The listing builds one solid part. Answer for the finished solid, in the listing's coordinates (mm). A direction names the side the tool comes from. Coordinates: 2 decimals unless noted, no trailing zeros. Write each loop counter-clockwise with the first axis right and the second up, starting at its lowest first coordinate (ties: lowest second). Pieces come first, ordered by that corner, then holes. Notation, with made-up numbers: M 58,17 L 79,17 A22 cw 79,42 Z; hole C -26.75,71.25 d4. An arc over 180 degrees is marked long. Write item = value, one per line. Start each with the question number.
```python
from build123d import *

# Parameters (mm, degrees)
F1_DEPTH = 6.35
F3_DEPTH = 2.54


with BuildPart() as f1:
    # F0 (on Top) → F1 (new body)
    with BuildSketch(Plane.XY):
        Polygon((-19.068402, 7.360227), (-42.225117, 7.360227), (-57.954384, -14.267517), (-20.852379, -14.267517), (-20.852379, -24.618464), (10.865408, -24.618464), (10.865408, -14.267517), (39.400437, -14.267517), (52.040033, 7.360227), (12.264185, 7.360227), (12.264185, 17.065071), (-19.068402, 17.065071), align=None)
    extrude(amount=F1_DEPTH)

    # F2 (on face) → F3 (join)
    with BuildSketch(Plane.XY.offset(6.35)):
        Polygon((-19.068402, 7.360227), (-42.225117, 7.360227), (-57.954384, -14.267517), (-20.852379, -14.267517), (-20.852379, -24.618464), (10.865408, -24.618464), (10.865408, -14.267517), (39.400437, -14.267517), (52.040033, 7.360227), (12.264185, 7.360227), (12.264185, 17.065071), (-19.068402, 17.065071), align=None)
        Polygon((-15.004402, 3.296227), (-15.004402, 13.001071), (8.200185, 13.001071), (8.200185, 3.296227), (44.957841, 3.296227), (37.068377, -10.203517), (6.801408, -10.203517), (6.801408, -20.554464), (-16.788379, -20.554464), (-16.788379, -10.203517), (-49.973623, -10.203517), (-40.155628, 3.296227), align=None, mode=Mode.SUBTRACT)
    extrude(amount=F3_DEPTH)


solid = f1.part
```
1. Straight lines are drawn through the part: L1, parallel to X at y = 7.5, z = 8.25; L2, parallel to Y at x = -21.5, z = 7; L3, parallel to Y at x = -19, z = 7. For each, find the intervals that lie inside material, in ascending order. Write a range as [from, to].
2. For faces 1 (the face through (45.63, -3.61, 4.38)), 2 (the face through (-33, -10.204, 8)), 3 (the face through (-40, -14.268, 4)), determine the directions among +Z, -Z, +X, -X, +Y, -Y from which every point of the face is accessible in a straight line to the end or side of a thin tool.
3. For a pull along Y with two mould halves and no side action, classify faces 4 (the face through (32, 7.36, 4)), 5 (the face through (-4, 13.001, 8)), 6 (the face through (12.264, 12, 4)) as pulls with the +Y half, pulls with the -Y half, needs draft (parallel to the pull), parting line crosses it, or undercut.
4. The part is cut by section C-C, the plane x = 16. Write down the section's boundary in (y, z).
5. The part is cut by section B-B, the plane z = 3. Write down the section's boundary in (x, y).
6. Each of these flat-tipped pins is pushed along its axis until it touches: pin 1 (2.5 mm diameter, centred on y = 12, z = 4.5, fed in from +X); pin 2 (2.5 mm diameter, centred on y = -20.5, z = 6, fed in from -X); pin 3 (2 mm diameter, centred on y = 7, z = 7.5, fed in from -X). Where does it stop, or does it pass through?
7. The part is cut by section A-A, the plane y = -15.5. Write down the section's boundary in (x, z), and give its area (3 significant figures).
Solution:
q1.L1 = [-19.07, -15], [8.2, 12.26]
q1.L2 = [-14.27, -10.2], [3.3, 7.36]
q1.L3 = [-24.62, -10.2], [3.3, 17.07]
q2.face_1 = +Z, -Z, +X, -Y
q2.face_2 = +Z
q2.face_3 = +Z, -Z, -X, -Y
q3.face_4 = pulls with the +Y half
q3.face_5 = undercut
q3.face_6 = needs draft
q4.outline = M -14.27,0 L 7.36,0 L 7.36,8.89 L 3.3,8.89 L 3.3,6.35 L -10.2,6.35 L -10.2,8.89 L -14.27,8.89 Z
q5.outline = M -57.95,-14.27 L -20.85,-14.27 L -20.85,-24.62 L 10.87,-24.62 L 10.87,-14.27 L 39.4,-14.27 L 52.04,7.36 L 12.26,7.36 L 12.26,17.07 L -19.07,17.07 L -19.07,7.36 L -42.23,7.36 Z
q6.pin_1 = 12.26
q6.pin_2 = -20.85
q6.pin_3 = -43.21
q7.outline = M -20.85,0 L 10.87,0 L 10.87,8.89 L 6.8,8.89 L 6.8,6.35 L -16.79,6.35 L -16.79,8.89 L -20.85,8.89 Z
q7.area = 222 mm^2
